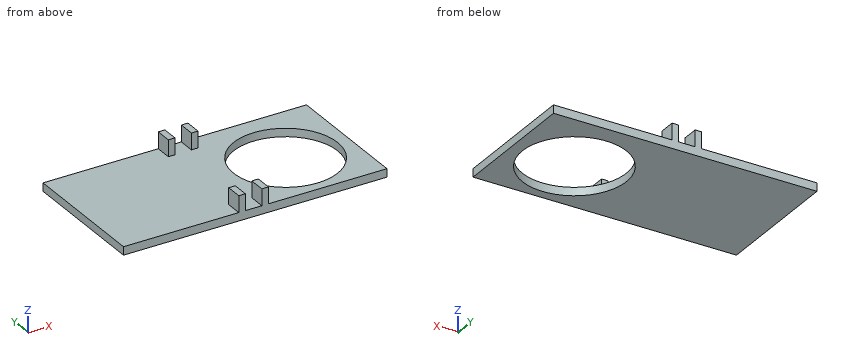
```python
from build123d import *

# Parameters (mm, degrees)
F0_W     = 203.2
F0_H     = 101.6
F0_R     = 40.12907
F1_DEPTH = 6.35
F2_W     = 5.08
F2_H     = 12.7
F3_DEPTH = 12.7
F4_DEPTH = 12.7


with BuildPart() as f1:
    # F0 (on Top) → F1 (new body)
    with BuildSketch(Plane.XY):
        with Locations((23.723893, -32.59281)):
            Rectangle(F0_W, F0_H)
        with Locations((76.090291, -35.990499)):
            Circle(F0_R, mode=Mode.SUBTRACT)
    extrude(amount=F1_DEPTH)

    # F2 (on face) → F3 (join)
    with BuildSketch(Plane.XY.offset(6.35)):
        with Locations((13.563893, -77.04281)):
            Rectangle(F2_W, F2_H)
        with Locations((31.343893, -77.04281)):
            Rectangle(F2_W, F2_H)
    extrude(amount=F3_DEPTH)

    # F2 (on face) → F4 (join)
    with BuildSketch(Plane.XY.offset(6.35)):
        with Locations((31.343893, -77.04281)):
            Rectangle(F2_W, F2_H)
        with Locations((13.563893, -77.04281)):
            Rectangle(F2_W, F2_H)
        with Locations((31.343893, 11.85719)):
            Rectangle(F2_W, F2_H)
        with Locations((13.563893, 11.85719)):
            Rectangle(F2_W, F2_H)
    extrude(amount=F4_DEPTH)


solid = f1.part
```
For this review, take the finished solid that the model builds, in its own axes (mm). Coordinates: 2 decimals unless noted, no trailing zeros. Loops run counter-clockwise (first coordinate to the right, second up) from the corner with the lowest first, then second, coordinate; pieces in that order, holes last.
1. Add section B-B, the plane y = -59. Give the boundary of the cut face in (x, z), then the cut area to 3 significant figures.
2. Add section D-D, the plane x = -22. Give the boundary of the cut face in (y, z).
3. For line 1 (X direction, y = 9.5, z = 8.25); line 2 (Y direction, x = 11.5, z = 9.5); line 3 (Z direction, x = -12, y = -14.5), list the stretches that pass through material, from the lowest coordinate up.
4. Insertion check: P1, Ø10, axis at y = 14.5, z = 14, coming from the +X side; P2, Ø1, axis at y = -69.5, z = 10.5, coming from the -X side; P3, Ø6.5, axis at y = -79, z = 15, coming from the -X side. Each pin has a flat end and moves straight along its axis. Give the tip position at first contact, or say it passes through.
5. Add section C-C, the plane x = 43.5. Give the boundary of the cut face in (y, z), then the cut area to 3 significant figures.
6. Add section A-A, the plane z = 12.5. Give the boundary of the cut face in (x, y), then the cut area to 3 significant figures.
Result:
1. outline: (-77.88, 0) - (43.21, 0) - (43.21, 6.35) - (-77.88, 6.35) - close; (108.97, 0) - (125.32, 0) - (125.32, 6.35) - (108.97, 6.35) - close
1. area: 873 mm2
2. outline: (-83.39, 0) - (18.21, 0) - (18.21, 6.35) - (-83.39, 6.35) - close
3. line 1: x = 11.02 to 16.1, 28.8 to 33.88
3. line 2: y = -83.39 to -70.69, 5.51 to 18.21
3. line 3: z = 0 to 6.35
4. P1: stops at x = 33.88
4. P2: passes through
4. P3: stops at x = 11.02
5. outline: (-83.39, 0) - (-59.4, 0) - (-59.4, 6.35) - (-83.39, 6.35) - close; (-12.58, 0) - (18.21, 0) - (18.21, 6.35) - (-12.58, 6.35) - close
5. area: 348 mm2
6. outline: (11.02, -83.39) - (16.1, -83.39) - (16.1, -70.69) - (11.02, -70.69) - close; (11.02, 5.51) - (16.1, 5.51) - (16.1, 18.21) - (11.02, 18.21) - close; (28.8, -83.39) - (33.88, -83.39) - (33.88, -70.69) - (28.8, -70.69) - close; (28.8, 5.51) - (33.88, 5.51) - (33.88, 18.21) - (28.8, 18.21) - close
6. area: 258 mm2
